```python
from build123d import *

# Parameters (mm, degrees)
BOSS_EXTRUDE1_DEPTH = 2
SKETCH2_W           = 4
SKETCH2_H           = 4
BOSS_EXTRUDE2_DEPTH = 10
SKETCH4_W           = 4
SKETCH4_H           = 4
BOSS_EXTRUDE4_DEPTH = 13
SKETCH5_W           = 4
SKETCH5_H           = 4
BOSS_EXTRUDE5_DEPTH = 25
FILLET2_R           = 2


with BuildPart() as part:
    # Sketch1 → Boss-Extrude1 (new, symmetric)
    with BuildSketch(Plane.XY):
        with BuildLine():
            Line((-7.1, -12.4), (-7.1, 12.4))
            ThreePointArc((-7.1, 12.4), (0, 19.5), (7.1, 12.4))
            Line((7.1, 12.4), (7.1, -12.4))
            ThreePointArc((7.1, -12.4), (0, -19.5), (-7.1, -12.4))
        make_face()
        with BuildLine():
            Line((-4.1, -12.4), (-4.1, 12.4))
            ThreePointArc((-4.1, 12.4), (0, 16.5), (4.1, 12.4))
            Line((4.1, 12.4), (4.1, -12.4))
            ThreePointArc((4.1, -12.4), (0, -16.5), (-4.1, -12.4))
        make_face(mode=Mode.SUBTRACT)
    extrude(amount=BOSS_EXTRUDE1_DEPTH, both=True)

    # Sketch2 → Boss-Extrude2 (add)
    with BuildSketch(Plane(origin=(7.1, 0, 0), x_dir=(0, 0, -1), z_dir=(1, 0, 0))):
        Rectangle(SKETCH2_W, SKETCH2_H)
    boss_extrude2 = extrude(amount=BOSS_EXTRUDE2_DEPTH)

    # Sketch4 → Boss-Extrude4 (add)
    with BuildSketch(Plane.XZ.offset(2)):
        with Locations((15.1, 0)):
            Rectangle(SKETCH4_W, SKETCH4_H)
    boss_extrude4 = extrude(amount=BOSS_EXTRUDE4_DEPTH)

    # Sketch5 → Boss-Extrude5 (add)
    with BuildSketch(Plane(origin=(17.1, 0, 0), x_dir=(0, 0, -1), z_dir=(1, 0, 0))):
        with Locations((0, -13)):
            Rectangle(SKETCH5_W, SKETCH5_H)
    boss_extrude5 = extrude(amount=BOSS_EXTRUDE5_DEPTH)

    # Mirror2: Boss-Extrude2, Boss-Extrude4, Boss-Extrude5 across plane
    add(boss_extrude2.mirror(Plane(origin=(0, 0, 0), x_dir=(0, 0, 1), z_dir=(1, 0, 0))))
    add(boss_extrude4.mirror(Plane(origin=(0, 0, 0), x_dir=(0, 0, 1), z_dir=(1, 0, 0))))
    add(boss_extrude5.mirror(Plane(origin=(0, 0, 0), x_dir=(0, 0, 1), z_dir=(1, 0, 0))))

    # Fillet2
    fillet2_edges = [part.edges().sort_by_distance(p)[0] for p in [
        (7.1, 2, 0),
        (7.1, -2, 0),
        (17.1, 2, 0),
        (13.1, -2, 0),
        (13.1, -15, 0),
        (17.1, -11, 0),
        (-17.1, 2, 0),
        (-7.1, 2, 0),
        (-7.1, -2, 0),
        (-13.1, -15, 0),
        (-13.1, -2, 0),
        (-17.1, -11, 0),
    ]]
    fillet(fillet2_edges, radius=FILLET2_R)


solid = part.part
```
For this review, take the finished solid that the model builds, in its own axes (mm). A direction names the side the tool comes from. Give positions to 0.01 mm unless a question says otherwise; leave off trailing zeros. Write each loop counter-clockwise with the first axis right and the second up, starting at its lowest first coordinate (ties: lowest second). Pieces come first, ordered by that corner, then holes.
Item 1: The part is to be moulded in two halves that separate along Y. For faces 1 (the face through (10, -2, 0)), 2 (the face through (-0.16, 19.5, 0.03)), 3 (the face through (0.1, -16.5, 0)), say which applies: +Y half, -Y half, draft (parallel to the pull), parting line (faces both ways), or undercut.
Item 2: Machinability: for faces 4 (the face through (-7.1, 8, 0)), 5 (the face through (-4.1, 0, 0)), 6 (the face through (30, -11, 0)), which of the approach directions +Z, -Z, +X, -X, +Y, -Y give a long, thin tool a straight path to every point of the face, cutting with its end or side? Answer none if there is none.
Item 3: Insertion check: P1, Ø2, axis at y = 8.5, z = -1, coming from the +X side; P2, Ø1.2, axis at y = 6.5, z = 1, coming from the -X side; P3, Ø1.2, axis at y = -6.5, z = 0.5, coming from the +X side. Each pin has a flat end and moves straight along its axis. Give the tip position at first contact, or say it passes through.
Item 4: Take a section at C-C (x = 28). Give the boundary of the cut face in (y, z).
Item 5: Wall thickness on probe 1 along X at (y, z) = (-12, 1); probe 2 along X at (y, z) = (4, -1.3); probe 3 along Y at (x, z) = (-1, 1.8): over which ranges is each line inside the solid? List them lowest first.
Item 6: Take a section at B-B (y = -3). Give the boundary of the cut face in (x, z).
Item 7: Take a section at A-A (x = 0). Give the boundary of the cut face in (y, z), and give its area (3 significant figures).
Established:
1. face 1: -Y half
1. face 2: +Y half
1. face 3: undercut
2. face 4: +Z, -Z, -X, +Y
2. face 5: +Z, -Z
2. face 6: +Z, -Z, +X, +Y
3. P1: stops at x = 7.1
3. P2: stops at x = -7.1
3. P3: stops at x = 17.1
4. outline: (-15, -2) - (-11, -2) - (-11, 2) - (-15, 2) - close
5. probe 1: x = -42.1 to -13.1, -7.1 to -4.1, 4.1 to 7.1, 13.1 to 42.1
5. probe 2: x = -7.1 to -4.1, 4.1 to 7.1
5. probe 3: y = -19.43 to -16.38, 16.38 to 19.43
6. outline: (-17.1, -2) - (-12.83, -2) - (-12.83, 2) - (-17.1, 2) - close; (-7.37, -2) - (-4.1, -2) - (-4.1, 2) - (-7.37, 2) - close; (4.1, -2) - (7.37, -2) - (7.37, 2) - (4.1, 2) - close; (12.83, -2) - (17.1, -2) - (17.1, 2) - (12.83, 2) - close
7. outline: (-19.5, -2) - (-16.5, -2) - (-16.5, 2) - (-19.5, 2) - close; (16.5, -2) - (19.5, -2) - (19.5, 2) - (16.5, 2) - close
7. area: 24.0 mm2
